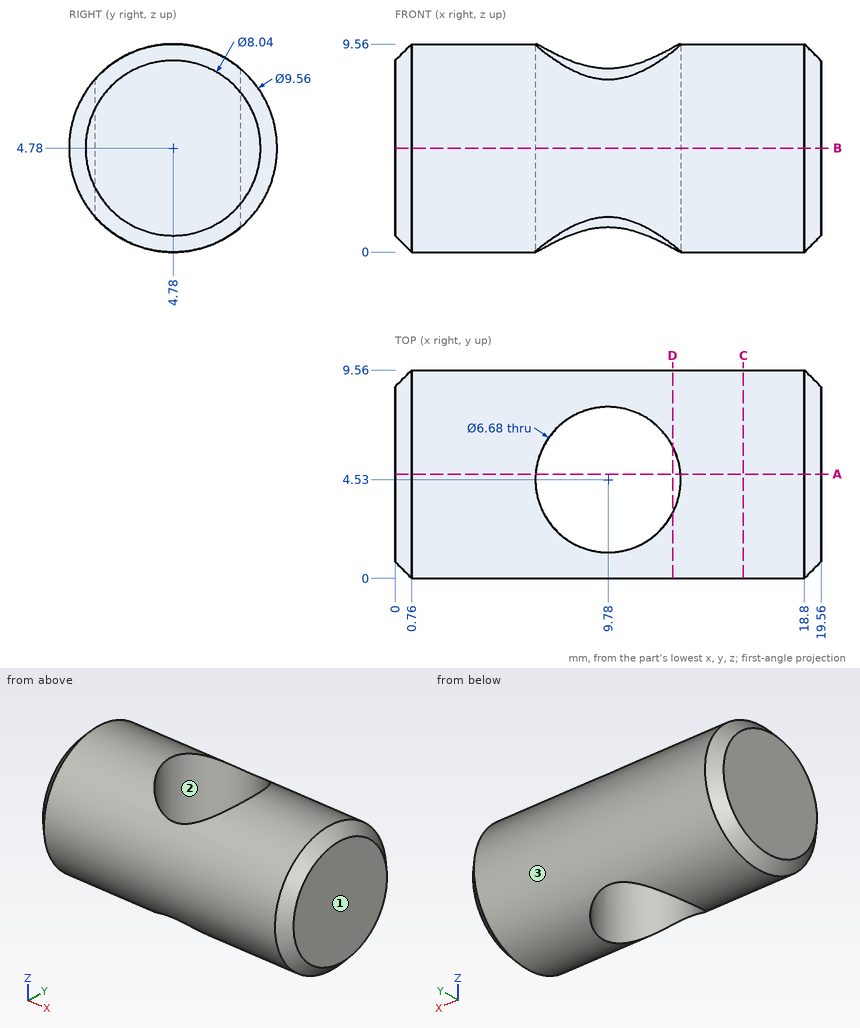
Study the drawing (mm; zero at the part's minimum x, y, z) and answer. Round coordinates to 2 decimals unless told otherwise and drop trailing zeros. Order: outer loops, then holes, each group sorted by start corner. A loop starts at its lowest first (then second) coordinate and runs counter-clockwise, first axis right, second up. Notation, with made-up numbers: M 53.25,6.5 L 71.25,6.5 A19 ccw 71.25,31.5 Z; hole C -17,64.5 d3. An arc over 180 degrees is marked long. One line per item, written item: value.
Q1. Find section A-A on y = 4.78. Write down the section's boundary in (x, z).
Derived:
outline: M 0,0.76 L 0.76,0 L 6.45,0 L 6.45,9.56 L 0.76,9.56 L 0,8.8 Z; M 13.11,0 L 18.8,0 L 19.56,0.76 L 19.56,8.8 L 18.8,9.56 L 13.11,9.56 Z
Q2. Find section C-C on x = 16. Write down the section's boundary in (y, z), then the cut area to 3 significant figures.
Derived:
outline: C 4.78,4.78 d9.56
area: 71.8 mm²
Q3. Determine the mould class of the marked faces 1, 2 and 3 for opening direction Y: released by +Y, released by -Y, zero draft, split by the parting line, or undercut.
Derived:
face 1: zero draft
face 2: undercut
face 3: split by the parting line
Q4. Find section B-B on z = 4.78. Write down the section's boundary in (x, y).
Derived:
outline: M 0,0.76 L 0.76,0 L 18.8,0 L 19.56,0.76 L 19.56,8.8 L 18.8,9.56 L 0.76,9.56 L 0,8.8 Z; hole C 9.78,4.53 d6.68
Q5. Find section D-D on x = 12.75. Write down the section's boundary in (y, z), then the cut area to 3 significant figures.
Derived:
outline: M 3,0.34 L 3,9.22 A4.78 ccw Z; M 6.06,0.17 A4.78 ccw 6.06,9.39 Z
area: 43.1 mm²
Q6. Straight lines are drawn through the part: line 1 (X direction, y = 4.53, z = 6.25); line 2 (Y direction, x = 9.78, z = 3.5); line 3 (X direction, y = 3.5, z = 7). For each, find the intervals that lie inside material, in ascending order.
Derived:
line 1: 0 to 6.44, 13.12 to 19.56
line 2: 0.17 to 1.19, 7.87 to 9.39
line 3: 0 to 6.6, 12.96 to 19.56
